```python
from build123d import *

# Parameters (mm, degrees)
F1_DEPTH = 50.8
F3_DEPTH = 12.7
F4_W     = 45.7905011984
F4_H     = 101.6
F4_R     = 12.307725437
F4_R_2   = 8.8836456499
F5_DEPTH = 25.4
F7_D     = 6.35


with BuildPart() as f1:
    # F0 (on Top) → F1 (new body, symmetric)
    with BuildSketch(Plane.XY):
        Polygon((25.4, -38.1), (0, 0), (-25.4, -38.1), align=None)
    extrude(amount=F1_DEPTH, both=True)

    # F2 (on face) → F3 (join, symmetric)
    with BuildSketch(Plane(origin=(0, 0, 0), x_dir=(-0.5547001962, -0.8320502943, 0), z_dir=(-0.8320502943, 0.5547001962, 0))):
        Polygon((45.7905011984, -1.1443360425), (0.0787186434, 15.7506404887), (8.4762908518, -33.2957603969), (45.7905011984, -2.2995244172), align=None)
    extrude(amount=F3_DEPTH, both=True)

    # F4 (on face) → F5 (join)
    with BuildSketch(Plane(origin=(0, 0, 0), x_dir=(-0.5547001962, 0.8320502943, 0), z_dir=(0.8320502943, 0.5547001962, 0))):
        with Locations((-22.8952505992, 0)):
            Rectangle(F4_W, F4_H)
        with Locations((-26.547158137, -29.2638558894)):
            Circle(F4_R, mode=Mode.SUBTRACT)
        with Locations((-24.961175397, -4.7561856918)):
            Circle(F4_R_2, mode=Mode.SUBTRACT)
        Polygon((-13.7583333333, -14.695818583), (-13.7583333333, 13.8239461095), (-0.2046684728, 15.7506404887), align=None, mode=Mode.SUBTRACT)
        with Locations((-26.547158137, -29.2638558894)):
            Circle(F4_R)
        with Locations((-24.961175397, -4.7561856918)):
            Circle(F4_R_2)
    extrude(amount=F5_DEPTH)

    # F7 (through all)
    with Locations(Plane(origin=(21.1340774762, 14.0893849841, 0), x_dir=(-0.5547001962, 0.8320502943, 0), z_dir=(0.8320502943, 0.5547001962, 0))):
        with Locations((-21.0971944034, 17.6605209708)):
            Hole(F7_D / 2)


solid = f1.part
```
Check sheet for the modelled part. Datum: model origin and axes. Units: mm. A direction names the side the tool comes from. Coordinates: 2 decimals unless noted, no trailing zeros. Order: outer loops, then holes, each group sorted by start corner. A loop starts at its lowest first (then second) coordinate and runs counter-clockwise, first axis right, second up. Notation, with made-up numbers: (-35.75, -24) -> (15.25, -24) arc R12 cw to (15.25, -12) -> close; hole circle Ø9 at (80.25, 13.25). An arc over 180 degrees is marked (long way). Write item = value, one per line. Start each with the question number.
1) Cross-section at B-B (y = 9). Enter the section's corners in (x, z).
2) Go/stop test with flat-tipped pins: P1, Ø3, axis at x = 31.5, z = 4.5, coming from the -Y side; P2, Ø4, axis at x = 5, z = 16.5, coming from the +Y side; P3, Ø12, axis at x = 22, z = -14, coming from the -Y side. Record where each tip stops, or that it passes through.
3) Cross-section at D-D (z = 22.5). Enter the section's corners in (x, y), then the cut area to 3 significant figures.
4) Material ranges on L1, parallel to Y at x = 12, z = 19.5; L2, parallel to Y at x = 4, z = -46; L3, parallel to X at y = -8, z = 2.5, recorded low to high.
5) Mould release check, pull along Y, two halves, no side actions. Record for faces 1 (the flat face through (12, -20, -50.8)), 2 (the flat face through (10.419, 6.946, -0.711)), 3 (the flat face through (-20.264, -18.787, -18.015)): +Y half, -Y half, draft (parallel to the pull), parting line (faces both ways), or undercut.
6) Cross-section at A-A (z = 4). Enter the section's corners in (x, y).
7) Cross-section at C-C (x = 19). State how many separate pieces and enclosed holes the cut face has, then the cut area to 3 significant figures.
8) Access from +Z, -Z, +X, -X, +Y, -Y to the whole of each face (thin tool, end or side, straight path). Record for faces 4 (the flat face through (14.239, 1.216, 0.741)), 5 (the flat face through (12, -20, 50.8)), 6 (the flat face through (-7.698, 0.061, -8.429)).
Ans:
q1.outline = (13.5, -50.8) -> (24.53, -50.8) -> (24.53, 2.47) -> (13.87, 15.75) -> (24.53, 14.91) -> (24.53, 50.8) -> (13.5, 50.8) -> close
q2.P1 = -35.03
q2.P2 = 4.67
q2.P3 = -38.1
q3.outline = (-25.4, -38.1) -> (25.4, -38.1) -> (46.53, -24.01) -> (21.13, 14.09) -> (0, 0) -> close
q3.area = 2,130 mm²
q4.L1 = -38.1 to -20.47, -14.25 to 8
q4.L2 = -38.1 to 2.67
q4.L3 = -20.6 to 7.77, 12.8 to 35.86
q5.face_1 = draft
q5.face_2 = +Y half
q5.face_3 = undercut
q6.outline = (-28.25, -19.47) -> (-17.68, -26.52) -> (-25.4, -38.1) -> (25.4, -38.1) -> (46.53, -24.01) -> (28.77, 2.64) -> (7.63, -11.45) -> (9.41, -8.78) -> (3.02, -4.52) -> (24.15, 9.57) -> (21.13, 14.09) -> (0, 0) -> (-1.16, -1.74) -> (-11.73, 5.31) -> close
q7.separate_pieces = 1
q7.enclosed_holes = 2
q7.area = 4,890 mm²
q8.face_4 = none
q8.face_5 = +Z, +X, -X, +Y, -Y
q8.face_6 = -Z, +Y
